For this review, take the finished solid that the model builds, in its own axes (mm). A direction names the side the tool comes from. Give positions to 0.01 mm unless a question says otherwise; leave off trailing zeros. Loops run counter-clockwise (first coordinate to the right, second up) from the corner with the lowest first, then second, coordinate; pieces in that order, holes last.
```python
from build123d import *

# Parameters (mm, degrees)
CROQUIS1_W              = 144
CROQUIS1_H              = 82
SALIENTE_EXTRUIR1_DEPTH = 2
CROQUIS3_W              = 8
CROQUIS3_H              = 45
SALIENTE_EXTRUIR2_DEPTH = 2
CROQUIS2_R              = 4
CROQUIS2_R_2            = 1.25
SALIENTE_EXTRUIR3_DEPTH = 7
CORTAR_EXTRUIR1_REACH   = 92.167
CROQUIS4_W              = 19
CROQUIS4_H              = 6
CORTAR_EXTRUIR2_REACH   = 92.167
CROQUIS5_R              = 1.75
CROQUIS7_W              = 19
CROQUIS7_H              = 3
SALIENTE_EXTRUIR4_DEPTH = 23
CORTAR_EXTRUIR3_REACH   = 113.808
CROQUIS9_R              = 1.75
NERVIO1_REACH           = 141.524
CROQUIS10_WALL_W        = 292.3620914
CROQUIS10_WALL_H        = 2
NERVIO2_START           = -2
NERVIO2_DEPTH           = 2
NERVIO3_REACH           = 149.061
CROQUIS12_WALL_W        = 307.43613199
CROQUIS12_WALL_H        = 2
NERVIO4_START           = -2
NERVIO4_DEPTH           = 2


# Read off the part's stored shape, not the designer's step: Nervio2, Nervio4
with BuildPart() as part:
    # Croquis1 → Saliente-Extruir1 (new body)
    with BuildSketch(Plane(origin=(0, 0, 0), x_dir=(1, 0, 0), z_dir=(0, 1, 0))):
        Rectangle(CROQUIS1_W, CROQUIS1_H)
    extrude(amount=SALIENTE_EXTRUIR1_DEPTH)

    # Croquis3 → Saliente-Extruir2 (add)
    with BuildSketch(Plane(origin=(0, 2, 0), x_dir=(1, 0, 0), z_dir=(0, 1, 0))):
        with Locations((-76, -18.5)):
            Rectangle(CROQUIS3_W, CROQUIS3_H)
    extrude(amount=-SALIENTE_EXTRUIR2_DEPTH)

    # Croquis2 → Saliente-Extruir3 (add)
    # profile 1 of 4: a face of its own
    with BuildSketch(Plane(origin=(0, 2, 0), x_dir=(1, 0, 0), z_dir=(0, 1, 0))):
        with Locations(Location((54, -27, 0), (0, 0, 270))):
            Circle(CROQUIS2_R)
        with Locations(Location((54, -27, 0), (0, 0, 270))):
            Circle(CROQUIS2_R_2, mode=Mode.SUBTRACT)
    # profile 2 of 4: a face of its own
    with BuildSketch(Plane(origin=(0, 2, 0), x_dir=(1, 0, 0), z_dir=(0, 1, 0))):
        with Locations(Location((5, -4, 0), (0, 0, 270))):
            Circle(CROQUIS2_R)
        with Locations(Location((5, -4, 0), (0, 0, 270))):
            Circle(CROQUIS2_R_2, mode=Mode.SUBTRACT)
    # profile 3 of 4: a face of its own
    with BuildSketch(Plane(origin=(0, 2, 0), x_dir=(1, 0, 0), z_dir=(0, 1, 0))):
        with Locations(Location((-24, -27, 0), (0, 0, 270))):
            Circle(CROQUIS2_R)
        with Locations(Location((-24, -27, 0), (0, 0, 270))):
            Circle(CROQUIS2_R_2, mode=Mode.SUBTRACT)
    # profile 4 of 4: a face of its own
    with BuildSketch(Plane(origin=(0, 2, 0), x_dir=(1, 0, 0), z_dir=(0, 1, 0))):
        with Locations(Location((-73, -4, 0), (0, 0, 270))):
            Circle(CROQUIS2_R)
        with Locations(Location((-73, -4, 0), (0, 0, 270))):
            Circle(CROQUIS2_R_2, mode=Mode.SUBTRACT)
    extrude(amount=SALIENTE_EXTRUIR3_DEPTH)

    # Croquis4 → Cortar-Extruir1 (cut, up to next)
    with BuildSketch(Plane(origin=(0, 2, 0), x_dir=(1, 0, 0), z_dir=(0, 1, 0)), mode=Mode.PRIVATE) as cortar_extruir1_sk1:
        with Locations((-49.5, -26)):
            Rectangle(CROQUIS4_W, CROQUIS4_H)
    cortar_extruir1_tool1 = extrude(cortar_extruir1_sk1.sketch, amount=-CORTAR_EXTRUIR1_REACH, mode=Mode.PRIVATE) & part.part
    # Croquis4 → Cortar-Extruir1 (cut, up to next)
    with BuildSketch(Plane(origin=(0, 2, 0), x_dir=(1, 0, 0), z_dir=(0, 1, 0)), mode=Mode.PRIVATE) as cortar_extruir1_sk2:
        with Locations((37.5, -26)):
            Rectangle(CROQUIS4_W, CROQUIS4_H)
    cortar_extruir1_tool2 = extrude(cortar_extruir1_sk2.sketch, amount=-CORTAR_EXTRUIR1_REACH, mode=Mode.PRIVATE) & part.part
    add(cortar_extruir1_tool1.solids().sort_by_distance((-49.5, 2, 26))[0], mode=Mode.SUBTRACT)
    add(cortar_extruir1_tool2.solids().sort_by_distance((37.5, 2, 26))[0], mode=Mode.SUBTRACT)

    # Croquis5 → Cortar-Extruir2 (cut, up to next)
    with BuildSketch(Plane(origin=(0, 2, 0), x_dir=(1, 0, 0), z_dir=(0, 1, 0)), mode=Mode.PRIVATE) as cortar_extruir2_sk1:
        with Locations(Location((-43.4, 25, 0), (0, 0, 270))):
            Circle(CROQUIS5_R)
    cortar_extruir2_tool1 = extrude(cortar_extruir2_sk1.sketch, amount=-CORTAR_EXTRUIR2_REACH, mode=Mode.PRIVATE) & part.part
    # Croquis5 → Cortar-Extruir2 (cut, up to next)
    with BuildSketch(Plane(origin=(0, 2, 0), x_dir=(1, 0, 0), z_dir=(0, 1, 0)), mode=Mode.PRIVATE) as cortar_extruir2_sk2:
        with Locations(Location((43.4, 25, 0), (0, 0, 270))):
            Circle(CROQUIS5_R)
    cortar_extruir2_tool2 = extrude(cortar_extruir2_sk2.sketch, amount=-CORTAR_EXTRUIR2_REACH, mode=Mode.PRIVATE) & part.part
    add(cortar_extruir2_tool1.solids().sort_by_distance((-43.4, 2, -25))[0], mode=Mode.SUBTRACT)
    add(cortar_extruir2_tool2.solids().sort_by_distance((43.4, 2, -25))[0], mode=Mode.SUBTRACT)

    # Croquis7 → Saliente-Extruir4 (add)
    with BuildSketch(Plane(origin=(0, 2, 0), x_dir=(1, 0, 0), z_dir=(0, 1, 0))):
        with Locations((-49.5, -31.5)):
            Rectangle(CROQUIS7_W, CROQUIS7_H)
        with Locations((49.5, -31.5)):
            Rectangle(CROQUIS7_W, CROQUIS7_H)
    extrude(amount=SALIENTE_EXTRUIR4_DEPTH)

    # Croquis9 → Cortar-Extruir3 (cut, up to next)
    with BuildSketch(Plane.XY.offset(33), mode=Mode.PRIVATE) as cortar_extruir3_sk1:
        with Locations((-54.5, 22)):
            Circle(CROQUIS9_R)
    cortar_extruir3_tool1 = extrude(cortar_extruir3_sk1.sketch, amount=-CORTAR_EXTRUIR3_REACH, mode=Mode.PRIVATE) & part.part
    # Croquis9 → Cortar-Extruir3 (cut, up to next)
    with BuildSketch(Plane.XY.offset(33), mode=Mode.PRIVATE) as cortar_extruir3_sk2:
        with Locations((-44.5, 22)):
            Circle(CROQUIS9_R)
    cortar_extruir3_tool2 = extrude(cortar_extruir3_sk2.sketch, amount=-CORTAR_EXTRUIR3_REACH, mode=Mode.PRIVATE) & part.part
    # Croquis9 → Cortar-Extruir3 (cut, up to next)
    with BuildSketch(Plane.XY.offset(33), mode=Mode.PRIVATE) as cortar_extruir3_sk3:
        with Locations((44.5, 22)):
            Circle(CROQUIS9_R)
    cortar_extruir3_tool3 = extrude(cortar_extruir3_sk3.sketch, amount=-CORTAR_EXTRUIR3_REACH, mode=Mode.PRIVATE) & part.part
    # Croquis9 → Cortar-Extruir3 (cut, up to next)
    with BuildSketch(Plane.XY.offset(33), mode=Mode.PRIVATE) as cortar_extruir3_sk4:
        with Locations((54.5, 22)):
            Circle(CROQUIS9_R)
    cortar_extruir3_tool4 = extrude(cortar_extruir3_sk4.sketch, amount=-CORTAR_EXTRUIR3_REACH, mode=Mode.PRIVATE) & part.part
    add(cortar_extruir3_tool1.solids().sort_by_distance((-54.5, 22, 33))[0], mode=Mode.SUBTRACT)
    add(cortar_extruir3_tool2.solids().sort_by_distance((-44.5, 22, 33))[0], mode=Mode.SUBTRACT)
    add(cortar_extruir3_tool3.solids().sort_by_distance((44.5, 22, 33))[0], mode=Mode.SUBTRACT)
    add(cortar_extruir3_tool4.solids().sort_by_distance((54.5, 22, 33))[0], mode=Mode.SUBTRACT)

    # Croquis10 wall → Nervio1 (add, up to next)
    with BuildSketch(Plane(origin=(-59, 6, 37), x_dir=(0, 0.707106781187, -0.707106781187), z_dir=(0, -0.707106781187, -0.707106781187)), mode=Mode.PRIVATE) as nervio1_sk1:
        with Locations((0, 1)):
            Rectangle(CROQUIS10_WALL_W, CROQUIS10_WALL_H)
    nervio1_tool1 = extrude(nervio1_sk1.sketch, amount=NERVIO1_REACH, mode=Mode.PRIVATE) - part.part
    add(nervio1_tool1.solids().sort_by_distance((-59, 6, 37))[0])

    # Nervio2 outline → Nervio2 (add)
    with BuildSketch(Plane(origin=(-40, 0, 0), x_dir=(0, 0, -1), z_dir=(1, 0, 0)).offset(NERVIO2_START)):
        Polygon((-33, 10), (-41, 2), (-33, 2), align=None)
    extrude(amount=NERVIO2_DEPTH)

    # Croquis12 wall → Nervio3 (add, up to next)
    with BuildSketch(Plane(origin=(59, 6, 37), x_dir=(0, -0.707106781187, 0.707106781187), z_dir=(0, -0.707106781187, -0.707106781187)), mode=Mode.PRIVATE) as nervio3_sk1:
        with Locations((0, 1)):
            Rectangle(CROQUIS12_WALL_W, CROQUIS12_WALL_H)
    nervio3_tool1 = extrude(nervio3_sk1.sketch, amount=NERVIO3_REACH, mode=Mode.PRIVATE) - part.part
    add(nervio3_tool1.solids().sort_by_distance((59, 6, 37))[0])

    # Nervio4 outline → Nervio4 (add)
    with BuildSketch(Plane.ZY.offset(-40).offset(NERVIO4_START)):
        Polygon((41, 2), (33, 10), (33, 2), align=None)
    extrude(amount=NERVIO4_DEPTH)


solid = part.part
```
Item 1: Clearance check with flat-ended pins moving along their axes: pin 1 Ø3 at (x, z) = (-24, 27) entering from +Y; pin 2 Ø9.5 at (x, y) = (-47.5, 8.5) entering from -Z; pin 3 Ø1 at (x, y) = (-27.5, 3) entering from +Z; pin 4 Ø8 at (x, z) = (27.5, 32) entering from -Y. State where each tip first meets the part, or that it passes through.
Answer:
pin 1: stops at y = 9
pin 2: stops at z = 30
pin 3: stops at z = 29.65
pin 4: stops at y = 0
Item 2: Tool access review of faces 4 (the flat face through (-40, 11, 32)), 5 (the flat face through (-50, 13, 30)), 6 (the cylindrical face through (-21.3, 5.45, 24.05)), 7 (the flat face through (53, 9, 26)), 8 (the flat face through (-42, 4, 35)): name each direction out of +Z, -Z, +X, -X, +Y, -Y from which nothing blocks a thin tool from reaching the whole face with its end or side.
Answer:
face 4: +Z, -Z, +Y
face 5: -Z, -X, +Y
face 6: +Y
face 7: -Z, +X, -X, +Y
face 8: +Z, +Y
Item 3: Take a section at A-A on y = 17.25. Give the boundary of the cut face in (x, z), and give its area (3 significant figures).
Answer:
outline: (-59, 30) - (-40, 30) - (-40, 33) - (-59, 33) - close; (40, 30) - (59, 30) - (59, 33) - (40, 33) - close
area: 114 mm2
Item 4: The part is to be moulded in two halves that separate along X. For faces 1 (the flat face through (49, 13, 33)), 2 (the flat face through (-59, 10.5, 32.6)), 3 (the flat face through (-58, 6, 37)), say which applies: released by +X, released by -X, zero draft, split by the parting line, or undercut.
Answer:
face 1: undercut
face 2: released by -X
face 3: zero draft
Item 5: For L1, parallel to X at y = 5, z = 27; L2, parallel to X at y = 13, z = 31; L3, parallel to Y at x = 15, z = -25.5, list the stretches that pass through material, from the lowest coordinate up.
Answer:
L1: x = -28 to -25.25, -22.75 to -20, 50 to 52.75, 55.25 to 58
L2: x = -59 to -40, 40 to 59
L3: y = 0 to 2
Item 6: Take a section at C-C on x = 21.5. Give the boundary of the cut face in (y, z).
Answer:
outline: (0, -41) - (2, -41) - (2, 41) - (0, 41) - close
Item 7: Take a section at B-B on x = -48.5. Give the boundary of the cut face in (y, z).
Answer:
outline: (0, -41) - (2, -41) - (2, 23) - (0, 23) - close; (0, 29) - (2, 29) - (2, 30) - (25, 30) - (25, 33) - (2, 33) - (2, 41) - (0, 41) - close
